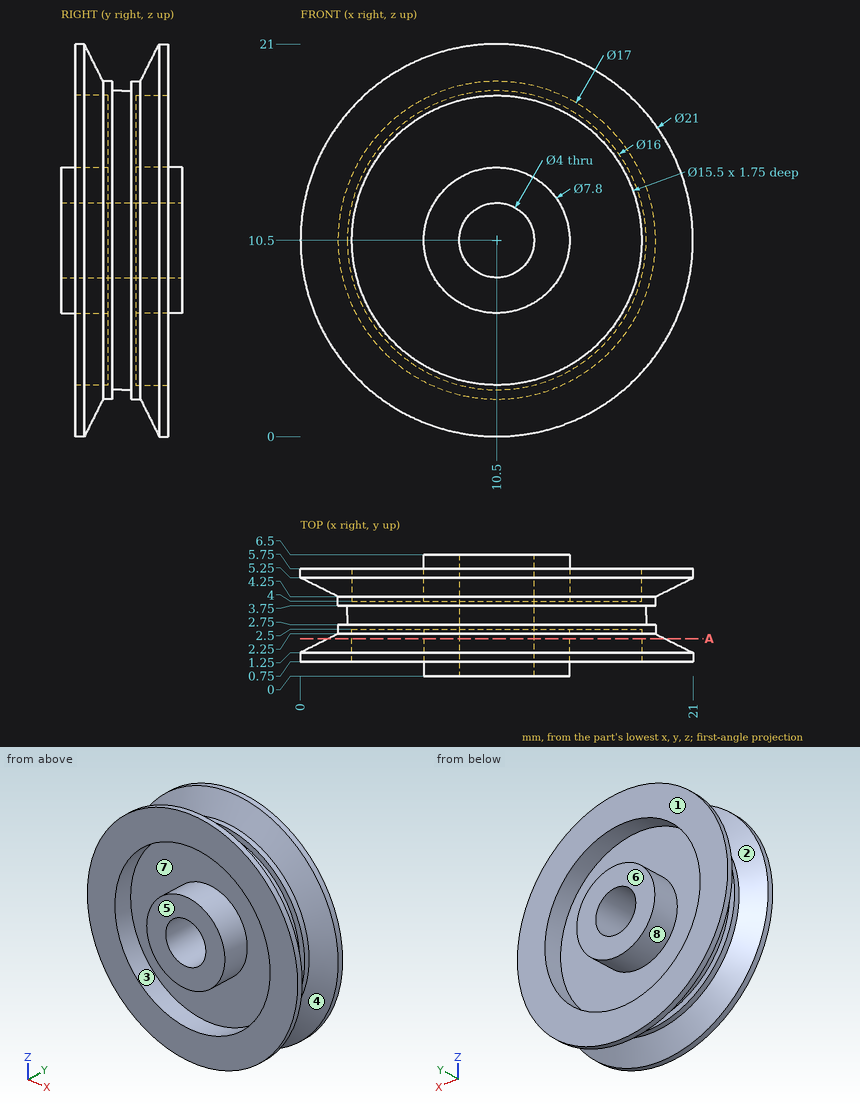
Geometry: see drawing. Coordinates: mm, zero at the bounding-box minimum. A direction names the side the tool comes from. Coordinates: 2 decimals unless noted, no trailing zeros. Order: outer loops, then holes, each group sorted by start corner. A loop starts at its lowest first (then second) coordinate and runs counter-clockwise, first axis right, second up. Notation, with made-up numbers: (-28.75, 66) - (-24.75, 66) arc R7 ccw to (-24.75, 77) - close; hole circle Ø1 at (22, -17.5). An arc over 180 degrees is marked (long way). Use one line per item in the form item = value.
1) Mould query, pull axis Z, two halves, no side actions, for the marked faces 1, 2 and 3. Classes: +Z half, -Z half, draft (parallel to the pull), parting line (faces both ways), or undercut.
Solutions:
face_1 = draft
face_2 = parting line
face_3 = undercut
2) Set-up query: the marked faces 4, 5, 6, 7 and 8. Return all of +Z, -Z, +X, -X, +Y, -Y with unobstructed straight access to the full face (end or side cutting, diameter ignored); none if empty.
Solutions:
face_4 = none
face_5 = +Z, -Z, +X, -X, -Y
face_6 = +Z, -Z, +X, -X, +Y
face_7 = -Y
face_8 = +Y
3) Ray query, L1, parallel to Z at x = 10.5, y = 1.2; L2, parallel to Z at x = 10.5, y = 4.95; L3, parallel to Z at x = 13.5, y = 1.5. Return the intervals inside material, ascending.
Solutions:
L1 = 0 to 2.75, 6.6 to 8.5, 12.5 to 14.4, 18.25 to 21
L2 = 0.6 to 2.75, 6.6 to 8.5, 12.5 to 14.4, 18.25 to 20.4
L3 = 0.96 to 3.35, 8.01 to 12.99, 17.65 to 20.04
4) Section A-A (y = 2). Return loops of the section in (x, z).
Solutions:
outline = circle Ø18 at (10.5, 10.5); circle Ø7.8 at (10.5, 10.5); hole circle Ø15.5 at (10.5, 10.5); hole circle Ø4 at (10.5, 10.5)
5) Pin query (flat end, axial travel): pin 1 (8.5 mm diameter, centred on x = 11.5, z = 10, fed in from +Y); pin 2 (8 mm diameter, centred on x = 18, z = 14, fed in from -Y); pin 3 (2 mm diameter, centred on x = 12, y = 5, fed in from +Z); pin 4 (3.5 mm diameter, centred on x = 10.5, z = 10.5, fed in from -Y). Return the tip coordinate at first contact, or that it passes through.
Solutions:
pin_1 = 6.5
pin_2 = 0.75
pin_3 = 20.99
pin_4 = through
